Can you work these out from the model? Positions are in its coordinate system, mm. Give positions to 0.01 mm unless a question says otherwise; leave off trailing zeros. Order: outer loops, then holes, each group sorted by start corner. A loop starts at its lowest first (then second) coordinate and runs counter-clockwise, first axis right, second up. Notation, with made-up numbers: M 43.5,-2.75 L 90.5,-2.75 A15 ccw 90.5,18.25 Z; hole C -7.5,-3.5 d1. An arc over 180 degrees is marked long. Answer as a JSON object with one key per item and string values.
```python
from build123d import *

# Parameters (mm, degrees)
SKETCH1_R                                           = 196.85
SKETCH1_R_2                                         = 107.95
SKETCH1_R_3                                         = 2.6289
SKETCH1_R_4                                         = 3.175
BOSS_EXTRUDE1_DEPTH                                 = 6.35
SKETCH3_R                                           = 204.7875
SKETCH3_R_2                                         = 196.85
BOSS_EXTRUDE2_DEPTH                                 = 6.35
CSK_FOR_1_4_FLAT_HEAD_MACHINE_SCREW_100_D           = 6.7564
CSK_FOR_1_4_FLAT_HEAD_MACHINE_SCREW_100_DEPTH       = 25.4
CSK_FOR_1_4_FLAT_HEAD_MACHINE_SCREW_100_CSINK_D     = 12.8778
CSK_FOR_1_4_FLAT_HEAD_MACHINE_SCREW_100_CSINK_ANGLE = 100
CSK_FOR_1_4_FLAT_HEAD_MACHINE_SCREW_100_TIP         = 2.029827343
SKETCH10_R                                          = 2.0193
CUT_EXTRUDE1_DEPTH                                  = 7.3500001


with BuildPart() as part:
    # Sketch1 → Boss-Extrude1 (new body)
    with BuildSketch(Plane(origin=(0, 0, 0), x_dir=(1, 0, 0), z_dir=(0, 1, 0))):
        Circle(SKETCH1_R)
        Circle(SKETCH1_R_2, mode=Mode.SUBTRACT)
        with Locations((69.85, -109.5375)):
            Circle(SKETCH1_R_3, mode=Mode.SUBTRACT)
        with Locations((69.85, -134.9375)):
            Circle(SKETCH1_R_3, mode=Mode.SUBTRACT)
        with Locations((101.6, -109.5375)):
            Circle(SKETCH1_R_3, mode=Mode.SUBTRACT)
        with Locations((101.6, -134.9375)):
            Circle(SKETCH1_R_3, mode=Mode.SUBTRACT)
        with Locations((101.6, 133.35)):
            Circle(SKETCH1_R_3, mode=Mode.SUBTRACT)
        with Locations((101.6, 158.75)):
            Circle(SKETCH1_R_3, mode=Mode.SUBTRACT)
        with Locations((133.35, -12.7)):
            Circle(SKETCH1_R_3, mode=Mode.SUBTRACT)
        with Locations((133.35, 12.7)):
            Circle(SKETCH1_R_3, mode=Mode.SUBTRACT)
        with Locations((-69.85, -134.9375)):
            Circle(SKETCH1_R_3, mode=Mode.SUBTRACT)
        with Locations((-101.6, -134.9375)):
            Circle(SKETCH1_R_3, mode=Mode.SUBTRACT)
        with Locations((-101.6, -109.5375)):
            Circle(SKETCH1_R_3, mode=Mode.SUBTRACT)
        with Locations((-69.85, -109.5375)):
            Circle(SKETCH1_R_3, mode=Mode.SUBTRACT)
        with Locations((-133.35, -12.7)):
            Circle(SKETCH1_R_3, mode=Mode.SUBTRACT)
        with Locations((-133.35, 12.7)):
            Circle(SKETCH1_R_3, mode=Mode.SUBTRACT)
        with Locations((-101.6, 158.75)):
            Circle(SKETCH1_R_3, mode=Mode.SUBTRACT)
        with Locations((-101.6, 133.35)):
            Circle(SKETCH1_R_3, mode=Mode.SUBTRACT)
        with Locations((0, 127)):
            Circle(SKETCH1_R_4, mode=Mode.SUBTRACT)
        with Locations((109.985226281, 63.5)):
            Circle(SKETCH1_R_4, mode=Mode.SUBTRACT)
        with Locations((109.985226281, -63.5)):
            Circle(SKETCH1_R_4, mode=Mode.SUBTRACT)
        with Locations((0, -127)):
            Circle(SKETCH1_R_4, mode=Mode.SUBTRACT)
        with Locations((-109.985226281, -63.5)):
            Circle(SKETCH1_R_4, mode=Mode.SUBTRACT)
        with Locations((-109.985226281, 63.5)):
            Circle(SKETCH1_R_4, mode=Mode.SUBTRACT)
    extrude(amount=BOSS_EXTRUDE1_DEPTH)

    # Sketch3 → Boss-Extrude2 (add)
    with BuildSketch(Plane(origin=(0, 6.35, 0), x_dir=(1, 0, 0), z_dir=(0, 1, 0))):
        Circle(SKETCH3_R)
        Circle(SKETCH3_R_2, mode=Mode.SUBTRACT)
    extrude(amount=-BOSS_EXTRUDE2_DEPTH)

    # CSK for 1/4 Flat Head Machine Screw (100)1
    with Locations(Plane(origin=(0, 6.35, 0), x_dir=(1, 0, 0), z_dir=(0, 1, 0))):
        with Locations((0, 127), (-109.985226281, 63.5), (-109.985226281, -63.5), (0, -127), (109.985226281, -60.325), (109.985226281, 63.5)):
            CounterSinkHole(CSK_FOR_1_4_FLAT_HEAD_MACHINE_SCREW_100_D / 2, CSK_FOR_1_4_FLAT_HEAD_MACHINE_SCREW_100_CSINK_D / 2, depth=CSK_FOR_1_4_FLAT_HEAD_MACHINE_SCREW_100_DEPTH, counter_sink_angle=CSK_FOR_1_4_FLAT_HEAD_MACHINE_SCREW_100_CSINK_ANGLE)
            with Locations((0, 0, -(CSK_FOR_1_4_FLAT_HEAD_MACHINE_SCREW_100_DEPTH + CSK_FOR_1_4_FLAT_HEAD_MACHINE_SCREW_100_TIP / 2))):  # 118° drill point
                Cone(0, CSK_FOR_1_4_FLAT_HEAD_MACHINE_SCREW_100_D / 2, CSK_FOR_1_4_FLAT_HEAD_MACHINE_SCREW_100_TIP, mode=Mode.SUBTRACT)

    # Sketch10 → Cut-Extrude1 (cut, through all)
    with BuildSketch(Plane(origin=(0, 6.35, 0), x_dir=(1, 0, 0), z_dir=(0, 1, 0))):
        with Locations((0, 200.025)):
            Circle(SKETCH10_R)
        with Locations((29.812179292, 197.790886016)):
            Circle(SKETCH10_R)
        with Locations((58.958403762, 191.138450477)):
            Circle(SKETCH10_R)
        with Locations((86.787594917, 180.216297802)):
            Circle(SKETCH10_R)
        with Locations((112.678094614, 165.268410833)):
            Circle(SKETCH10_R)
        with Locations((136.051551873, 146.628700663)):
            Circle(SKETCH10_R)
        with Locations((156.385842281, 124.713547617)):
            Circle(SKETCH10_R)
        with Locations((173.226731392, 100.0125)):
            Circle(SKETCH10_R)
        with Locations((186.198021573, 73.077338399)):
            Circle(SKETCH10_R)
        with Locations((195.009955634, 44.509749815)):
            Circle(SKETCH10_R)
        with Locations((199.465689531, 14.94788697)):
            Circle(SKETCH10_R)
        with Locations((199.465689531, -14.94788697)):
            Circle(SKETCH10_R)
        with Locations((195.009955634, -44.509749815)):
            Circle(SKETCH10_R)
        with Locations((186.198021573, -73.077338399)):
            Circle(SKETCH10_R)
        with Locations((173.226731392, -100.0125)):
            Circle(SKETCH10_R)
        with Locations((156.385842281, -124.713547617)):
            Circle(SKETCH10_R)
        with Locations((136.051551873, -146.628700663)):
            Circle(SKETCH10_R)
        with Locations((112.678094614, -165.268410833)):
            Circle(SKETCH10_R)
        with Locations((86.787594917, -180.216297802)):
            Circle(SKETCH10_R)
        with Locations((58.958403762, -191.138450477)):
            Circle(SKETCH10_R)
        with Locations((29.812179292, -197.790886016)):
            Circle(SKETCH10_R)
        with Locations((0, -200.025)):
            Circle(SKETCH10_R)
        with Locations((-29.812179292, -197.790886016)):
            Circle(SKETCH10_R)
        with Locations((-58.958403762, -191.138450477)):
            Circle(SKETCH10_R)
        with Locations((-86.787594917, -180.216297802)):
            Circle(SKETCH10_R)
        with Locations((-112.678094614, -165.268410833)):
            Circle(SKETCH10_R)
        with Locations((-136.051551873, -146.628700663)):
            Circle(SKETCH10_R)
        with Locations((-156.385842281, -124.713547617)):
            Circle(SKETCH10_R)
        with Locations((-173.226731392, -100.0125)):
            Circle(SKETCH10_R)
        with Locations((-186.198021573, -73.077338399)):
            Circle(SKETCH10_R)
        with Locations((-195.009955634, -44.509749815)):
            Circle(SKETCH10_R)
        with Locations((-199.465689531, -14.94788697)):
            Circle(SKETCH10_R)
        with Locations((-199.465689531, 14.94788697)):
            Circle(SKETCH10_R)
        with Locations((-195.009955634, 44.509749815)):
            Circle(SKETCH10_R)
        with Locations((-186.198021573, 73.077338399)):
            Circle(SKETCH10_R)
        with Locations((-173.226731392, 100.0125)):
            Circle(SKETCH10_R)
        with Locations((-156.385842281, 124.713547617)):
            Circle(SKETCH10_R)
        with Locations((-136.051551873, 146.628700663)):
            Circle(SKETCH10_R)
        with Locations((-112.678094614, 165.268410833)):
            Circle(SKETCH10_R)
        with Locations((-86.787594917, 180.216297802)):
            Circle(SKETCH10_R)
        with Locations((-58.958403762, 191.138450477)):
            Circle(SKETCH10_R)
        with Locations((-29.812179292, 197.790886016)):
            Circle(SKETCH10_R)
    extrude(amount=-CUT_EXTRUDE1_DEPTH, mode=Mode.SUBTRACT)


solid = part.part
```
1) Thinking about a two-plate mould opening in X: for faces 1 (the face through (88, 6.35, 88)), 2 (the face through (-79.56, 3.13, -72.96)), 3 (the face through (-113.243, 3.906, 64.851)), 4 (the face through (94.5, 3.22, 181.68)), which applies, pulls with the +X half, pulls with the -X half, needs draft (parallel to the pull), parting line crosses it, or undercut?
Results found:
{"face 1": "needs draft", "face 2": "undercut", "face 3": "undercut", "face 4": "parting line crosses it"}
2) I'm going to push flat-ended pins straight in: pin 1 Ø1.5 at (y, z) = (0.5, 28) entering from -X; pin 2 Ø1.5 at (y, z) = (1.5, -147.5) entering from -X; pin 3 Ø1.5 at (y, z) = (3, 75) entering from +X. Where does each tip first touch, or does it pass through?
Results found:
{"pin 1": "stops at x = -202.97", "pin 2": "stops at x = -142.84", "pin 3": "stops at x = 190.85"}
3) I want a section at A-A on z = 89. Write out the boundary of the cut face in (x, y).
Results found:
{"outline": "M -184.44,0 L -61.09,0 L -61.09,6.35 L -184.44,6.35 Z; M 61.09,0 L 184.44,0 L 184.44,6.35 L 61.09,6.35 Z"}
4) I want a section at B-B on y = 5. Count the separate pieces of the cut face and the enclosed holes in it, and give its area (3 significant figures).
Results found:
{"separate pieces": "1", "enclosed holes": "65", "area": "93,800 mm²"}
5) I need wall thicknesses on L1, parallel to X at y = 4.75, z = 4.5; L2, parallel to X at y = 1.75, z = -145.5; L3, parallel to X at y = 2, z = -1. Which ranges of each line are inside material? Lowest first, please.
Results found:
{"L1": "x = -204.74 to -107.86, 107.86 to 204.74", "L2": "x = -144.11 to -137.73, -134.38 to 134.38, 137.73 to 144.11", "L3": "x = -204.79 to -107.95, 107.95 to 204.79"}
